Work out the finished part from the listing and answer in its coordinate system (mm). A direction names the side the tool comes from. Give positions to 0.01 mm unless a question says otherwise; leave off trailing zeros. Loops run counter-clockwise (first coordinate to the right, second up) from the corner with the lowest first, then second, coordinate; pieces in that order, holes last.
```python
from build123d import *

# Parameters (mm, degrees)
F0_R     = 18.796
F1_DEPTH = 25.4
F3_DEPTH = 10.16
F5_DEPTH = 19.05
F6_R     = 4.445
F7_DEPTH = 31.497


with BuildPart() as f1:
    # F0 (on Top) → F1 (new body)
    with BuildSketch(Plane.XY):
        Circle(F0_R)
    extrude(amount=-F1_DEPTH)

    # F2 (on face) → F3 (cut)
    with BuildSketch(Plane(origin=(0, 0, -25.4), x_dir=(1, 0, 0), z_dir=(0, 0, -1))):
        with BuildLine():
            Line((13.856393, -12.7), (-13.856393, -12.7))
            ThreePointArc((-13.856393, -12.7), (0, -18.796), (13.856393, -12.7))
        make_face()
        with BuildLine():
            Line((-13.856393, 12.7), (13.856393, 12.7))
            ThreePointArc((13.856393, 12.7), (0, 18.796), (-13.856393, 12.7))
        make_face()
    extrude(amount=-F3_DEPTH, mode=Mode.SUBTRACT)

    # F4 (on face) → F5 (cut)
    with BuildSketch(Plane(origin=(0, 0, -25.4), x_dir=(1, 0, 0), z_dir=(0, 0, -1))):
        with BuildLine():
            Line((-6.35, 9.525), (-12.381035, 9.525))
            ThreePointArc((-12.381035, 9.525), (-15.621, 0), (-12.381035, -9.525))
            Line((-12.381035, -9.525), (-6.35, -9.525))
            Line((-6.35, -9.525), (-6.35, -3.81))
            Line((-6.35, -3.81), (6.35, -3.81))
            Line((6.35, -3.81), (6.35, -9.525))
            Line((6.35, -9.525), (12.381035, -9.525))
            ThreePointArc((12.381035, -9.525), (15.621, 0), (12.381035, 9.525))
            Line((12.381035, 9.525), (6.35, 9.525))
            Line((6.35, 9.525), (6.35, 3.81))
            Line((6.35, 3.81), (-6.35, 3.81))
            Line((-6.35, 3.81), (-6.35, 9.525))
        make_face()
    extrude(amount=-F5_DEPTH, mode=Mode.SUBTRACT)

    # F6 (on face) → F7 (cut, through all)
    with BuildSketch(Plane.XZ.offset(12.7)):
        with Locations((0, -20.32)):
            Circle(F6_R)
    extrude(amount=-F7_DEPTH, mode=Mode.SUBTRACT)


solid = f1.part
```
Q1. Section D-D on y = 0 is taken. Give the vertices of the cut face in (x, z), plus the area to 3 significant figures.
Q2. Determine the mould class of faces 5 (the face through (-0.96, -8.32, -24.66)), 6 (the face through (-9, 9.525, -16)), 7 (the face through (0, 0, 0)) for opening direction Z: +Z half, -Z half, draft (parallel to the pull), parting line (faces both ways), or undercut.
Q3. Section C-C on z = -20.32 is taken. Give the vertices of the cut face in (x, y) (3 decimals), plus the area to 3 significant figures.
Q4. Section A-A on z = -14.5 is taken. Give the vertices of the cut face in (x, y) (3 decimals), plus the area to 3 significant figures.
Q5. Consider line 1 along Z through (x, y) = (0, -10) (3 decimals); line 2 along X through (y, z) = (6, -21.25); line 3 along Y through (x, z) = (-10.5, -18.5) (3 decimals). Determine where each line is inside the solid, lowest interval first.
Q6. Given pin 1 (6.5 mm diameter, centred on y = 7, z = -17.5, fed in from +X); pin 2 (4 mm diameter, centred on x = 3, z = -14, fed in from +Y); pin 3 (11 mm diameter, centred on x = 3, z = -21, fed in from -Y); pin 4 (8 mm diameter, centred on x = 0, z = -20.32, fed in from -Y), each flat-ended and moving along its own axis, determine where each tip first touches the part or whether it passes through.
Q7. Which of the six approach directions +Z, -Z, +X, -X, +Y, -Y give full straight-line access (tool end or side, diameter ignored) to faces 1 (the face through (0, 12.7, -25)), 2 (the face through (6.35, 7, -16)), 3 (the face through (0, -15, -15.24)), 4 (the face through (8.673, -16.675, -9.7))?
Q8. Section B-B on x = 0 is taken. Give the vertices of the cut face in (y, z) (3 decimals).
Check result:
1. outline: (-18.8, -25.4) - (-15.62, -25.4) - (-15.62, -6.35) - (15.62, -6.35) - (15.62, -25.4) - (18.8, -25.4) - (18.8, 0) - (-18.8, 0) - close
1. area: 360 mm2
2. face 5: undercut
2. face 6: draft
2. face 7: +Z half
3. outline: (-13.856, -12.7) - (-4.445, -12.7) - (-4.445, -3.81) - (-6.35, -3.81) - (-6.35, -9.525) - (-12.381, -9.525) arc R15.621 cw to (-12.381, 9.525) - (-6.35, 9.525) - (-6.35, 3.81) - (-4.445, 3.81) - (-4.445, 12.7) - (-13.856, 12.7) arc R18.796 ccw to start; (4.445, -12.7) - (13.856, -12.7) arc R18.796 ccw to (13.856, 12.7) - (4.445, 12.7) - (4.445, 3.81) - (6.35, 3.81) - (6.35, 9.525) - (12.381, 9.525) arc R15.621 cw to (12.381, -9.525) - (6.35, -9.525) - (6.35, -3.81) - (4.445, -3.81) - close
3. area: 307 mm2
4. outline: circle Ø37.592 at (0, 0); hole (-12.381, -9.525) - (-6.35, -9.525) - (-6.35, -3.81) - (6.35, -3.81) - (6.35, -9.525) - (12.381, -9.525) arc R15.621 ccw to (12.381, 9.525) - (6.35, 9.525) - (6.35, 3.81) - (-6.35, 3.81) - (-6.35, 9.525) - (-12.381, 9.525) arc R15.621 ccw to start
4. area: 699 mm2
5. line 1: z = -25.4 to -24.765, -15.875 to 0
5. line 2: x = -17.81 to -14.42, -6.35 to -4.35, 4.35 to 6.35, 14.42 to 17.81
5. line 3: y = -12.7 to -9.525, 9.525 to 12.7
6. pin 1: stops at x = 18.42
6. pin 2: stops at y = 18.77
6. pin 3: stops at y = -12.7
6. pin 4: passes through
7. face 1: -Z, +X, -X, +Y
7. face 2: -Z
7. face 3: -Z, +X, -X, -Y
7. face 4: +Z, -Z
8. outline: (-18.796, -15.24) - (-12.7, -15.24) - (-12.7, -15.875) - (-3.81, -15.875) - (-3.81, -6.35) - (3.81, -6.35) - (3.81, -15.875) - (12.7, -15.875) - (12.7, -15.24) - (18.796, -15.24) - (18.796, 0) - (-18.796, 0) - close; (-12.7, -25.4) - (-3.81, -25.4) - (-3.81, -24.765) - (-12.7, -24.765) - close; (3.81, -25.4) - (12.7, -25.4) - (12.7, -24.765) - (3.81, -24.765) - close
